from build123d import *

# Parameters (mm, degrees)
F0_R      = 10
F1_DEPTH  = 10
F0_R_2    = 6
F2_DEPTH  = 20
F0_W      = 60
F0_H      = 20
F3_DEPTH  = 70
F4_R      = 16
F5_DEPTH  = 50
F6_R      = 3
F9_DEPTH  = 65.4
F10_DEPTH = 15
F11_DEPTH = 15
F12_R     = 5
F13_R     = 5


with BuildPart() as f1:
    # F0 (on Top) → F1 (new body)
    with BuildSketch(Plane.XY):
        with BuildLine():
            Line((-38.7446990098, 40), (-38.7446990098, 0))
            Line((-38.7446990098, 0), (21.2553009902, 0))
            Line((21.2553009902, 0), (21.2553009902, 40))
            ThreePointArc((21.2553009902, 40), (12.4685044258, 61.2132034356), (-8.7446990098, 70))
            ThreePointArc((-8.7446990098, 70), (-29.9579024454, 61.2132034356), (-38.7446990098, 40))
        make_face()
        with Locations((-8.7446990098, 40)):
            Circle(F0_R, mode=Mode.SUBTRACT)
    extrude(amount=F1_DEPTH)

    # F0 (on Top) → F2 (join)
    with BuildSketch(Plane.XY):
        with Locations((-8.7446990098, 40)):
            Circle(F0_R)
        with Locations((-8.7446990098, 40)):
            Circle(F0_R_2, mode=Mode.SUBTRACT)
    extrude(amount=F2_DEPTH)

    # F0 (on Top) → F3 (join)
    with BuildSketch(Plane.XY):
        with Locations((-8.7446990098, -10)):
            Rectangle(F0_W, F0_H)
    extrude(amount=F3_DEPTH)

    # F4 (on face) → F5 (join)
    with BuildSketch(Plane.XZ.offset(20)):
        with Locations((-8.7446990098, 35)):
            Circle(F4_R)
    extrude(amount=F5_DEPTH)

    # F6
    f6_edges = [f1.edges().sort_by_distance(p)[0] for p in [
        (-24.744699, -70, 35),
    ]]
    fillet(f6_edges, radius=F6_R)

    # F8 (on face) → F9 (cut)
    with BuildSketch(Plane(origin=(-38.7446990098, 0, 0), x_dir=(0, -1, 0), z_dir=(-1, 0, 0))):
        Polygon((10.7179676972, 70), (0, 70), (0, 30), align=None)
    extrude(amount=-F9_DEPTH, mode=Mode.SUBTRACT)

    # F8 (on face) → F10 (join)
    with BuildSketch(Plane(origin=(-38.7446990098, 0, 0), x_dir=(0, -1, 0), z_dir=(-1, 0, 0))):
        Polygon((10.7179676972, 70), (0, 30), (0, 10), (-40, 10), (-40, 0), (20, 0), (20, 70), align=None)
        Polygon((10.7179676972, 70), (0, 70), (0, 30), align=None)
    extrude(amount=-F10_DEPTH)

    # F7 (on face) → F11 (join)
    with BuildSketch(Plane.YZ.offset(21.2553009902)):
        Polygon((0, 10), (0, 30), (-10.7179676972, 70), (-20, 70), (-20, 0), (40, 0), (40, 10), align=None)
        Polygon((0, 30), (0, 70), (-10.7179676972, 70), align=None)
    extrude(amount=-F11_DEPTH)

    # F12
    f12_edges = [f1.edges().sort_by_distance(p)[0] for p in [
        (21.255301, -10, 70),
    ]]
    fillet(f12_edges, radius=F12_R)

    # F13
    f13_edges = [f1.edges().sort_by_distance(p)[0] for p in [
        (-38.744699, -10, 70),
    ]]
    fillet(f13_edges, radius=F13_R)


solid = f1.part
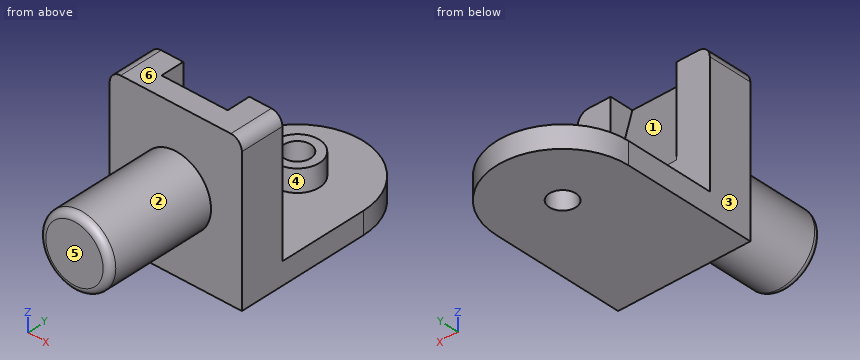
The listing builds one solid part. Answer for the finished solid, in the listing's coordinates (mm). Face numbers are marked on the shaded views. A direction names the side the tool comes from. Coordinates: 2 decimals unless noted, no trailing zeros. Order: outer loops, then holes, each group sorted by start corner. A loop starts at its lowest first (then second) coordinate and runs counter-clockwise, first axis right, second up. Notation, with made-up numbers: (50.25, -1) -> (72.25, -1) arc R6 cw to (72.25, 9) -> close; hole circle Ø5 at (-33, 13). An arc over 180 degrees is marked (long way). Answer in a Markdown table with one row per item. Add a question column.
Item 1: Find section B-B (z = 60.5). Write down the section's boundary in (x, y), then the cut area to 3 significant figures.
Item 2: Which of the six approach directions +Z, -Z, +X, -X, +Y, -Y give full straight-line access (tool end or side, diameter ignored) to the marked faces 1, 2 and 3?
Item 3: Find the intervals of material crossed by L1, parallel to Y at x = -24, z = 13.5; L2, parallel to Z at x = -31, y = 1; L3, parallel to Y at x = -11.5, z = 43.5, in increasing order. Write a range as from..to.
Item 4: Find section C-C (y = -58). Write down the section's boundary in (x, z).
Item 5: Determine the mould class of the marked faces 4, 5 and 6 for opening direction Y: +Y half, -Y half, draft (parallel to the pull), parting line (faces both ways), or undercut.
Item 6: Find section A-A (y = -4). Write down the section's boundary in (x, z).
Item 7: Find section D-D (z = 35). Write down the section's boundary in (x, y).
Item 8: Each of these flat-tipped pins is pushed along its axis until it touches: P1, Ø5, axis at x = -4, z = 52.5, coming from the -Y side; P2, Ø2, axis at x = -16, z = 35, coming from the +Y side; P3, Ø10, axis at x = -8.5, y = 39.5, coming from the +Z side; P4, Ø1, axis at x = -18, y = -45, coming from the -Z side. Where does it stop, or does it pass through?
Result set:
| question | item | result |
|---|---|---|
| 1 | outline | (-38.74, -20) -> (21.26, -20) -> (21.26, 0) -> (6.26, 0) -> (6.26, -8.17) -> (-23.74, -8.17) -> (-23.74, 0) -> (-38.74, 0) -> close |
| 1 | area | 955 mm² |
| 2 | face 1 | +Z, +Y |
| 2 | face 2 | -Y |
| 2 | face 3 | +Z, -Z, -X, +Y, -Y |
| 3 | L1 | y = -20..0 |
| 3 | L2 | z = 0..10 |
| 3 | L3 | y = -70..-3.62 |
| 4 | outline | circle Ø32 at (-8.74, 35) |
| 5 | face 4 | undercut |
| 5 | face 5 | -Y half |
| 5 | face 6 | draft |
| 6 | outline | (-38.74, 0) -> (21.26, 0) -> (21.26, 65) arc R5 ccw to (16.26, 70) -> (6.26, 70) -> (6.26, 44.93) -> (-23.74, 44.93) -> (-23.74, 70) -> (-33.74, 70) arc R5 ccw to (-38.74, 65) -> close |
| 7 | outline | (-38.74, -20) -> (-24.74, -20) -> (-24.74, -67) arc R3 ccw to (-21.74, -70) -> (4.26, -70) arc R3 ccw to (7.26, -67) -> (7.26, -20) -> (21.26, -20) -> (21.26, 0) -> (6.26, 0) -> (6.26, -1.34) -> (-23.74, -1.34) -> (-23.74, 0) -> (-38.74, 0) -> close |
| 8 | P1 | stops at y = -68.44 |
| 8 | P2 | stops at y = -1.07 |
| 8 | P3 | passes through |
| 8 | P4 | stops at z = 21.61 |
